Geometry check sheet. Reference: the model listing, model coordinates, mm. Face numbers are marked on the shaded views. A direction names the side the tool comes from. Round coordinates to 2 decimals unless told otherwise and drop trailing zeros. Order: outer loops, then holes, each group sorted by start corner. A loop starts at its lowest first (then second) coordinate and runs counter-clockwise, first axis right, second up.
(1) Thickness scan on L1, parallel to X at y = -88, z = -45; L2, parallel to Y at x = 26.5, z = 20.5; L3, parallel to Z at x = -34.5, y = -20. Record the ranges inside material, lowest first.
(2) Set-up check for the marked faces 1 and 2: record each of +Z, -Z, +X, -X, +Y, -Y from which the full face is reachable in a straight line by a thin tool's end or side.
(3) Cross-section at D-D on y = -64.5. Enter the section's corners in (x, z).
(4) Cross-section at B-B on y = -29. Enter the section's corners in (x, z), and give its area (3 significant figures).
(5) Gauge pin test, flat ends, axial feed: P1, Ø1.5, axis at x = -35.5, y = -80, coming from the +Z side; P2, Ø1.5, axis at y = -50, z = -6.5, coming from the -X side; P3, Ø4, axis at x = -4.5, z = -30.5, coming from the -Y side. Record the tip position at first contact, or that the pin passes through.
(6) Cross-section at C-C on z = 33. Enter the section's corners in (x, y), and give its area (3 significant figures).
(7) Cross-section at A-A on x = 6. Enter the section's corners in (y, z), and give its area (3 significant figures).
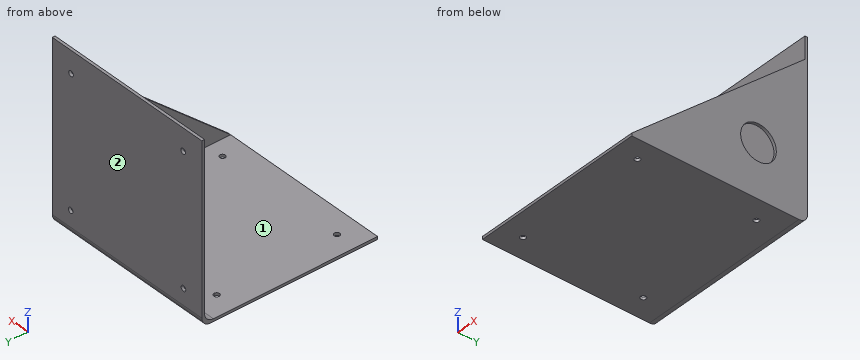
from build123d import *

# Parameters (mm, degrees)
F1_DEPTH  = 101.6
F0_W      = 50.8
F0_H      = 100.0125
F0_R      = 1.5875
F2_DEPTH  = 1.5875
F4_DEPTH  = 1.5875
F5_R      = 5.08
F6_R      = 5.08
F7_R      = 1.5875
F8_DEPTH  = 25.4
F10_R     = 10.3124
F11_DEPTH = 25.4


with BuildPart() as f1:
    # F0 (on Front) → F1 (new body)
    with BuildSketch(Plane.XZ):
        Polygon((-38.6839361429, -44.711994803), (-51.3839361429, -44.711994803), (-51.3839361429, -46.299494803), (50.2160638571, -46.299494803), (50.2160638571, -44.711994803), (-0.5839361429, -44.711994803), align=None)
    extrude(amount=F1_DEPTH)

    # F0 (on Front) → F2 (join)
    with BuildSketch(Plane.XZ):
        with BuildLine():
            Line((-38.6839361429, 55.300505197), (-51.3839361429, 55.300505197))
            Line((-51.3839361429, 55.300505197), (-51.3839361429, 42.600505197))
            Line((-51.3839361429, 42.600505197), (-40.2714361429, 42.600505197))
            ThreePointArc((-40.2714361429, 42.600505197), (-39.8064681581, 43.7230372122), (-38.6839361429, 44.188005197))
            Line((-38.6839361429, 44.188005197), (-38.6839361429, 55.300505197))
        make_face()
        with BuildLine():
            Line((-0.5839361429, 55.300505197), (-38.6839361429, 55.300505197))
            Line((-38.6839361429, 55.300505197), (-38.6839361429, 44.188005197))
            ThreePointArc((-38.6839361429, 44.188005197), (-37.5614041278, 43.7230372122), (-37.0964361429, 42.600505197))
            ThreePointArc((-37.0964361429, 42.600505197), (-38.6839361429, 41.013005197), (-40.2714361429, 42.600505197))
            Line((-40.2714361429, 42.600505197), (-51.3839361429, 42.600505197))
            Line((-51.3839361429, 42.600505197), (-51.3839361429, -44.711994803))
            Line((-51.3839361429, -44.711994803), (-38.6839361429, -44.711994803))
            Line((-38.6839361429, -44.711994803), (-0.5839361429, -44.711994803))
            Line((-0.5839361429, -44.711994803), (-0.5839361429, 55.300505197))
        make_face()
        with BuildLine():
            ThreePointArc((-37.3273452338, -32.01409415), (-37.7821543509, -33.1263745165), (-38.8859815975, -33.6013317316))
            ThreePointArc((-38.8859815975, -33.6013317316), (-40.0475361168, -30.9018137835), (-37.3273452338, -32.01409415))
        make_face(mode=Mode.SUBTRACT)
        with Locations((24.8160638571, 5.294255197)):
            Rectangle(F0_W, F0_H)
        with Locations((37.746972948, -32.01409415)):
            Circle(F0_R, mode=Mode.SUBTRACT)
        with Locations((37.5160638571, 42.600505197)):
            Circle(F0_R, mode=Mode.SUBTRACT)
        Polygon((-38.6839361429, -44.711994803), (-51.3839361429, -44.711994803), (-51.3839361429, -46.299494803), (50.2160638571, -46.299494803), (50.2160638571, -44.711994803), (-0.5839361429, -44.711994803), align=None)
    extrude(amount=F2_DEPTH)

    # F5
    f5_edges = [f1.edges().sort_by_distance(p)[0] for p in [
        (-0.583936, 0, -46.299495),
    ]]
    fillet(f5_edges, radius=F5_R)

    # F6
    f6_edges = [f1.edges().sort_by_distance(p)[0] for p in [
        (-0.583936, -1.5875, -44.711995),
    ]]
    fillet(f6_edges, radius=F6_R)

    # F7 (on face) → F8 (cut)
    with BuildSketch(Plane.XY.offset(-44.711994803)):
        with BuildLine():
            ThreePointArc((-38.6839361429, -17.78), (-39.8064681581, -20.4900320151), (-37.0964361429, -19.3675))
            ThreePointArc((-37.0964361429, -19.3675), (-37.5614041278, -18.2449679849), (-38.6839361429, -17.78))
        make_face()
        with Locations((-38.6839361429, -88.9)):
            Circle(F7_R)
        with Locations((37.6694120758, -18.8978454596)):
            Circle(F7_R)
        with Locations((38.5247778081, -88.4250840479)):
            Circle(F7_R)
    extrude(amount=-F8_DEPTH, mode=Mode.SUBTRACT)


with BuildPart() as f4:
    # F3 (on face) → F4 (new body)
    with BuildSketch(Plane.YZ.offset(50.2160638571)):
        Polygon((-1.5875, -44.711994803), (-1.5875, 42.600505197), (-101.6, -44.711994803), align=None)
    extrude(amount=-F4_DEPTH)

    # F9: union F1
    add(f1.part)

    # F10 (on face) → F11 (cut)
    with BuildSketch(Plane.YZ.offset(50.2160638571)):
        with Locations((-28.4118975516, -15.4491972514)):
            Circle(F10_R)
    extrude(amount=-F11_DEPTH, mode=Mode.SUBTRACT)


solid = f4.part
Found:
1. L1: x = -51.38 to -39.99, -37.38 to 37, 40.05 to 50.22
1. L2: y = -1.59 to 0
1. L3: z = -46.3 to -44.71
2. face 1: +Z, -X, -Y
2. face 2: +Z, -Z, +X, -X, +Y
3. outline: (-51.38, -46.3) - (50.22, -46.3) - (50.22, -12.32) - (48.63, -12.32) - (48.63, -44.71) - (-51.38, -44.71) - close
4. outline: (-51.38, -46.3) - (50.22, -46.3) - (50.22, -25.74) - (48.63, -25.74) - (48.63, -44.71) - (-51.38, -44.71) - close; (48.63, -5.15) - (50.22, -5.15) - (50.22, 18.67) - (48.63, 18.67) - close
4. area: 229 mm2
5. P1: stops at z = -44.71
5. P2: stops at x = 48.63
5. P3: stops at y = -1.59
6. outline: (-51.38, -1.59) - (48.63, -1.59) - (48.63, -12.58) - (50.22, -12.58) - (50.22, 0) - (-51.38, 0) - close
6. area: 179 mm2
7. outline: (-101.6, -46.3) - (-5.08, -46.3) arc R5.08 ccw to (0, -41.22) - (0, 55.3) - (-1.59, 55.3) - (-1.59, -39.63) arc R5.08 cw to (-6.67, -44.71) - (-101.6, -44.71) - close
7. area: 320 mm2
